Verification items for the finished model (mm, model axes). A direction names the side the tool comes from. Round coordinates to 2 decimals unless told otherwise and drop trailing zeros. Write each loop counter-clockwise with the first axis right and the second up, starting at its lowest first coordinate (ties: lowest second). Pieces come first, ordered by that corner, then holes. Notation, with made-up numbers: (3, 52.5) -> (50, 52.5) arc R20 ccw to (50, 81.5) -> close; hole circle Ø6 at (62, 88). An arc over 180 degrees is marked (long way). Use CSV: the item, a comma, the result in double quotes.
```python
from build123d import *

# Parameters (mm, degrees)
BOSS_EXTRUDE1_DEPTH = 48.26
CUT_EXTRUDE1_DEPTH  = 103.251
SKETCH3_R           = 1.905
CUT_EXTRUDE2_DEPTH  = 118.604958351


with BuildPart() as part:
    # Sketch1 → Boss-Extrude1 (new body)
    with BuildSketch(Plane(origin=(0, 0, 0), x_dir=(1, 0, 0), z_dir=(0, 1, 0))):
        with BuildLine():
            Line((-19.05, 99.798083649), (-19.764375, 103.540511786))
            ThreePointArc((-19.764375, 103.540511786), (0, 105.41), (19.764375, 103.540511786))
            Line((19.764375, 103.540511786), (19.05, 99.798083649))
            ThreePointArc((19.05, 99.798083649), (0, 101.6), (-19.05, 99.798083649))
        make_face()
    extrude(amount=BOSS_EXTRUDE1_DEPTH)

    # Sketch2 → Cut-Extrude1 (cut)
    with BuildSketch(Plane.XY):
        with BuildLine():
            Line((-2.54, 23.540829588), (-3.81, 25.786244382))
            Line((-3.81, 25.786244382), (-3.81, 48.26))
            Line((-3.81, 48.26), (-2.54, 48.26))
            Line((-2.54, 48.26), (-2.54, 27.152392088))
            Line((-2.54, 27.152392088), (-1.836175497, 25.908))
            Line((-1.836175497, 25.908), (1.776041068, 25.908))
            Line((1.776041068, 25.908), (2.54, 27.283126078))
            Line((2.54, 27.283126078), (2.54, 48.26))
            Line((2.54, 48.26), (3.81, 48.26))
            Line((3.81, 48.26), (3.81, 25.908))
            Line((3.81, 25.908), (2.505613998, 23.560105196))
            ThreePointArc((2.505613998, 23.560105196), (0.019710062, 13.890662649), (-2.54, 23.540829588))
        make_face()
    extrude(amount=-CUT_EXTRUDE1_DEPTH, mode=Mode.SUBTRACT)

    # Sketch3 → Cut-Extrude2 (cut, through all)
    with BuildSketch(Plane.XY):
        with Locations((-15.24, 44.45)):
            Circle(SKETCH3_R)
        with Locations((15.24, 44.45)):
            Circle(SKETCH3_R)
        with Locations((-15.24, 3.81)):
            Circle(SKETCH3_R)
        with Locations((15.24, 3.81)):
            Circle(SKETCH3_R)
    extrude(amount=-CUT_EXTRUDE2_DEPTH, mode=Mode.SUBTRACT)


solid = part.part
```
Q1. Section check D-D (y = 3.81). Record the cut outline in (x, z) (3 decimals).
Filled in:
outline,"(-19.764, -103.541) arc R105.41 ccw to (-17.145, -104.006) -> (-17.145, -100.143) arc R101.6 cw to (-19.05, -99.798) -> close; (-13.335, -104.563) arc R105.41 ccw to (13.335, -104.563) -> (13.335, -100.721) arc R101.6 cw to (-13.335, -100.721) -> close; (17.145, -104.006) arc R105.41 ccw to (19.764, -103.541) -> (19.05, -99.798) arc R101.6 cw to (17.145, -100.143) -> close"
Q2. Material ranges on L1, parallel to Y at x = -15.24, z = -103 (3 decimals); L2, parallel to X at y = 3.81, z = -102.8 (3 decimals); L3, parallel to Y at x = 0, z = -102.05, recorded low to high.
Filled in:
L1,"0 to 1.905, 5.715 to 42.545, 46.355 to 48.26"
L2,"-19.623 to -17.145, -13.335 to 13.335, 17.145 to 19.623"
L3,"0 to 13.89, 25.91 to 48.26"
Q3. Go/stop test with flat-tipped pins: P1, Ø9.5, axis at x = 0, y = 19.05, coming from the +Z side; P2, Ø4.5, axis at x = 15.24, y = 3.81, coming from the +Z side; P3, Ø10, axis at x = -13, y = 6, coming from the +Z side. Record where each tip stops, or that it passes through.
Filled in:
P1,"z = -103.25"
P2,"z = -100.08"
P3,"z = -99.99"
Q4. Section check A-A (x = -15.24). Record the cut outline in (y, z) (1 decimal), plus the area to 3 significant figures.
Filled in:
outline,"(0, -104.3) -> (1.9, -104.3) -> (1.9, -100.5) -> (0, -100.5) -> close; (5.7, -104.3) -> (42.5, -104.3) -> (42.5, -100.5) -> (5.7, -100.5) -> close; (46.4, -104.3) -> (48.3, -104.3) -> (48.3, -100.5) -> (46.4, -100.5) -> close"
area,"157 mm²"
Q5. Access from +Z, -Z, +X, -X, +Y, -Y to the whole of each face (thin tool, end or side, straight path). Record for faces 5 (the cylindrical face through (0, 36.9, -101.6)), 6 (the flat face through (3.81, 37, -102)), 7 (the flat face through (0, 25.908, -102)), 8 (the cylindrical face through (-0.28, 23.79, -105.41)), 9 (the cylindrical face through (13.84, 5.1, -102.32)).
Filled in:
face 5,"+Z, +Y, -Y"
face 6,"+Z, +Y"
face 7,"+Z"
face 8,"-Z, +Y, -Y"
face 9,"+Z, -Z"
Q6. Section check B-B (y = 19.05). Record the cut outline in (x, z).
Filled in:
outline,"(-19.76, -103.54) arc R105.41 ccw to (19.76, -103.54) -> (19.05, -99.8) arc R101.6 cw to (5.16, -101.47) -> (5.16, -103.25) -> (-5.16, -103.25) -> (-5.16, -101.47) arc R101.6 cw to (-19.05, -99.8) -> close"
Q7. Mould release check, pull along Y, two halves, no side actions. Record for faces 1 (the flat face through (-19.4, 23.79, -101.64)), 2 (the cylindrical face through (14.99, 46.34, -102.32)), 3 (the flat face through (0, 0, -103)), 4 (the cylindrical face through (-13.423, 4.382, -102.319)): released by +Y, released by -Y, zero draft, split by the parting line, or undercut.
Filled in:
face 1,"zero draft"
face 2,"undercut"
face 3,"released by -Y"
face 4,"undercut"
Q8. Section check C-C (x = 0). Record the cut outline in (y, z), plus the area to 3 significant figures.
Filled in:
outline,"(0, -105.41) -> (48.26, -105.41) -> (48.26, -101.6) -> (25.91, -101.6) -> (25.91, -103.25) -> (13.89, -103.25) -> (13.89, -101.6) -> (0, -101.6) -> close"
area,"164 mm²"
